Can you work these out from the model? Positions are in its coordinate system, mm. A direction names the side the tool comes from. Coordinates: 2 decimals unless noted, no trailing zeros. Write each loop counter-clockwise with the first axis right and the second up, starting at its lowest first coordinate (ties: lowest second). Pieces come first, ordered by that corner, then holes. Notation, with made-up numbers: (-26, 13) -> (18, 13) arc R32 cw to (18, 44) -> close; hole circle Ø1 at (66.25, 56.5). An arc over 180 degrees is marked (long way). Use one line per item in the form item = value.
Autodesk Inventor part; units mm, degrees
ref_plane "YZ Plane" through (0, 0, 0) normal (1, 0, 0) x (0, 1, 0)
ref_plane "XZ Plane" through (0, 0, 0) normal (0, 1, 0) x (-1, 0, 0)
ref_plane "XY Plane" through (0, 0, 0) normal (0, 0, 1) x (1, 0, 0)
sketch "Sketch1" plane through (0, 0, 0) normal (0, 0, 1) x (1, 0, 0)
  line L0 (0, 0) -> (15, 0)
  line L1 (15, 0) -> (15, 16)
  line L2 (15, 16) -> (0, 16)
  line L3 (0, 16) -> (0, 0)
  dimension "d0" = 15
  dimension "d1" = 16
extrude "Extrusion1" add sketch "Sketch1" along normal blind 17
sketch "Esquisse2" plane through (0, 0, 0) normal (0, 0, -1) x (-1, 0, 0)
  line L0 (0, 0) -> (-15, 0) construction
  line L1 (0, 16) -> (0, 0) construction
  line L2 (-15, 16) -> (0, 16) construction
  line L3 (-15, 0) -> (-15, 16) construction
  line L4 (-13.5, 15) -> (-1.5, 15)
  line L5 (-1.5, 15) -> (-1.5, 10)
  line L6 (-1.5, 10) -> (-13.5, 10)
  line L7 (-13.5, 10) -> (-13.5, 15)
  line L8 (-13.5, 6) -> (-1.5, 6)
  line L9 (-1.5, 6) -> (-1.5, 1)
  line L10 (-1.5, 1) -> (-13.5, 1)
  line L11 (-13.5, 1) -> (-13.5, 6)
  line L12 (-7.5, 0) -> (-7.5, 16) construction
  dimension "d4" = 12
  dimension "d5" = 5
  dimension "d6" = 5
  dimension "d7" = 1
  dimension "d8" = 4
extrude "Extrusion2" cut sketch "Esquisse2" against normal blind 15
properties part number "R001" material "Acier / Stahl"
Q1. For faces 1 (the flat face through (7, 1, 7)), 2 (the flat face through (8, 16, 8)), which set-ups out of +Z, -Z, +X, -X, +Y, -Y let a thin tool reach every point of the face, with its end or its side?
Return value:
face_1 = -Z
face_2 = +Z, -Z, +X, -X, +Y
Q2. If I drill on line 1 (Y direction, x = 10.75, z = 7.25); line 2 (X direction, y = 3.5, z = 2); line 3 (Z direction, x = 5, y = 5.5), over which ranges is the centre line in solid material (lowest first)? Write a range as from..to.
Return value:
line_1 = 0..1, 6..10, 15..16
line_2 = 0..1.5, 13.5..15
line_3 = 15..17
Q3. Suppose I cut it at A-A (z = 13). Write out the boundary of the cut face in (x, y), then the cut area to 3 significant figures.
Return value:
outline = (0, 0) -> (15, 0) -> (15, 16) -> (0, 16) -> close; hole (1.5, 1) -> (13.5, 1) -> (13.5, 6) -> (1.5, 6) -> close; hole (1.5, 10) -> (13.5, 10) -> (13.5, 15) -> (1.5, 15) -> close
area = 120 mm2
Q4. Will this pin go through, and if not, where does the flat tip stop? pin 1 (4 mm diameter, centred on x = 8.5, y = 12.5, fed in from -Z).
Return value:
pin_1 = 15
Q5. Suppose I cut it at C-C (y = 4.5). Write out the boundary of the cut face in (x, z), then the cut area to 3 significant figures.
Return value:
outline = (0, 0) -> (1.5, 0) -> (1.5, 15) -> (13.5, 15) -> (13.5, 0) -> (15, 0) -> (15, 17) -> (0, 17) -> close
area = 75.0 mm2
Q6. Suppose I cut it at B-B (x = 5.5). Write out the boundary of the cut face in (y, z).
Return value:
outline = (0, 0) -> (1, 0) -> (1, 15) -> (6, 15) -> (6, 0) -> (10, 0) -> (10, 15) -> (15, 15) -> (15, 0) -> (16, 0) -> (16, 17) -> (0, 17) -> close
Q7. Thinking about a two-plate mould opening in Y: for faces 3 (the flat face through (0, 8, 8)), 4 (the flat face through (7, 0, 8)), 5 (the flat face through (13.5, 12, 7)), 6 (the flat face through (1.5, 4, 7)), which applies, released by +Y, released by -Y, zero draft, split by the parting line, or undercut?
Return value:
face_3 = zero draft
face_4 = released by -Y
face_5 = undercut
face_6 = undercut
